Check sheet for the drawn part. Datum: minimum x, y, z corner. Units: mm. A direction names the side the tool comes from. Round coordinates to 2 decimals unless told otherwise and drop trailing zeros. Write each loop counter-clockwise with the first axis right and the second up, starting at its lowest first coordinate (ties: lowest second). Pieces come first, ordered by that corner, then holes. Notation, with made-up numbers: M -33,-20 L 11,-20 A35 cw 11,14 Z; hole C 40.5,72 d9. An arc over 180 degrees is marked long. Use a Markdown table: item, result.
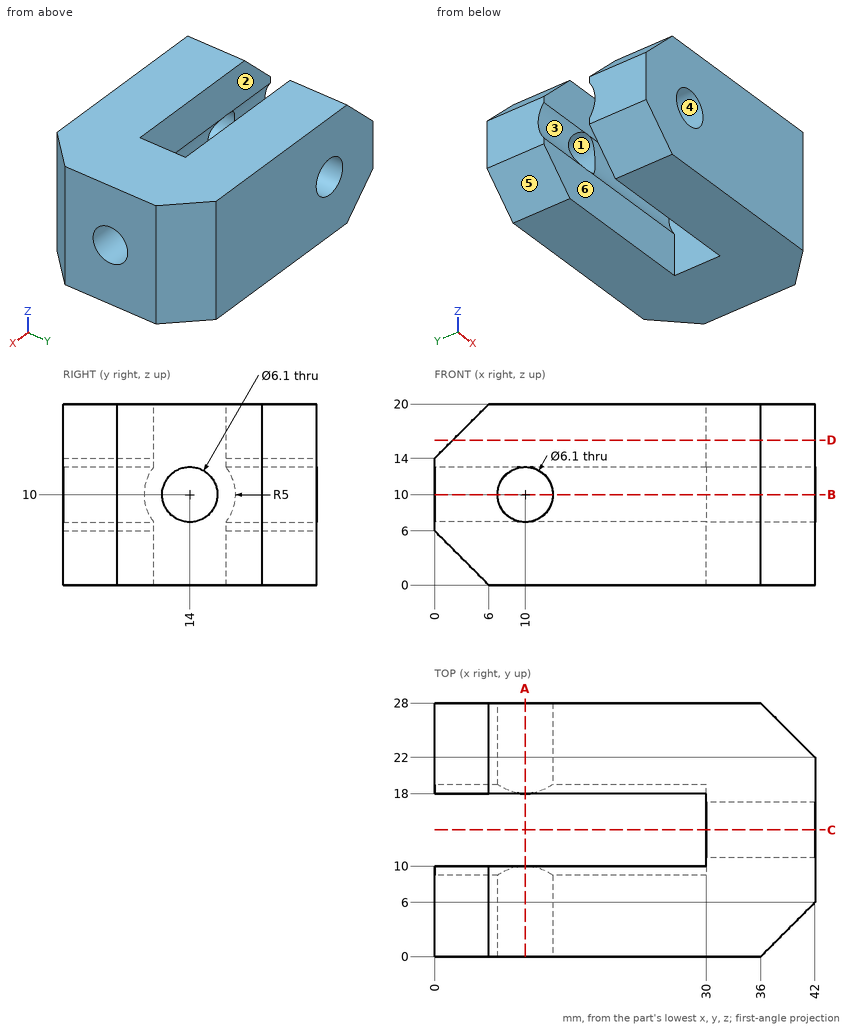
Item 1: Material ranges on line 1 along X through (y, z) = (21, 10); line 2 along Y through (x, z) = (25, 1.75); line 3 along Z through (x, y) = (10, 21.75), recorded low to high. Write a range as from..to.
Outcome:
| item | result |
|---|---|
| line 1 | x = 0..6.95, 13.05..42 |
| line 2 | y = 0..10, 18..28 |
| line 3 | z = 0..6.95, 13.05..20 |
Item 2: Cross-section at A-A, the plane x = 10. Record the cut outline in (y, z).
Outcome:
| item | result |
|---|---|
| outline | M 0,0 L 10,0 L 10,6.95 L 0,6.95 Z; M 0,13.05 L 10,13.05 L 10,20 L 0,20 Z; M 18,0 L 28,0 L 28,6.95 L 18,6.95 Z; M 18,13.05 L 28,13.05 L 28,20 L 18,20 Z |
Item 3: Go/stop test with a flat-tipped pin: pin 1 (3 mm diameter, centred on y = 15.5, z = 14, fed in from -X). Record where the tip stops, or that it passes through.
Outcome:
| item | result |
|---|---|
| pin 1 | stops at x = 30 |
Item 4: Mould release check, pull along X, two halves, no side actions. Record for the marked faces 4, 5 and 6: +X half, -X half, draft (parallel to the pull), parting line (faces both ways), or undercut.
Outcome:
| item | result |
|---|---|
| face 4 | undercut |
| face 5 | -X half |
| face 6 | draft |
Item 5: Cross-section at C-C, the plane y = 14. Record the cut outline in (x, z).
Outcome:
| item | result |
|---|---|
| outline | M 30,0 L 42,0 L 42,6.95 L 30,6.95 Z; M 30,13.05 L 42,13.05 L 42,20 L 30,20 Z |
Item 6: Cross-section at D-D, the plane z = 16. Record the cut outline in (x, y), and give its area (3 significant figures).
Outcome:
| item | result |
|---|---|
| outline | M 2,0 L 36,0 L 42,6 L 42,22 L 36,28 L 2,28 L 2,18 L 30,18 L 30,10 L 2,10 Z |
| area | 860 mm2 |
Item 7: Cross-section at B-B, the plane z = 10. Record the cut outline in (x, y).
Outcome:
| item | result |
|---|---|
| outline | M 0,0 L 6.95,0 L 6.95,9 L 0,9 Z; M 0,19 L 6.95,19 L 6.95,28 L 0,28 Z; M 13.05,0 L 36,0 L 42,6 L 42,10.95 L 30,10.95 L 30,9 L 13.05,9 Z; M 13.05,19 L 30,19 L 30,17.05 L 42,17.05 L 42,22 L 36,28 L 13.05,28 Z |
Item 8: Access from +Z, -Z, +X, -X, +Y, -Y to the whole of each face (thin tool, end or side, straight path). Record for the marked faces 1, 2 and 3.
Outcome:
| item | result |
|---|---|
| face 1 | +Y, -Y |
| face 2 | +Z, -Z, -X |
| face 3 | -X |
